```python
from build123d import *

# Parameters (mm, degrees)
SKETCH1_R           = 4.7625
BOSS_EXTRUDE1_DEPTH = 5.08
FILLET1_R           = 1.27


with BuildPart() as part:
    # Sketch1 → Boss-Extrude1 (new body)
    with BuildSketch(Plane.XY):
        Polygon((6.705982891, 2.965320691), (0.784948396, 7.290211886), (-5.921034494, 4.324891195), (-6.705982891, -2.965320691), (-0.784948396, -7.290211886), (5.921034494, -4.324891195), align=None)
        Circle(SKETCH1_R, mode=Mode.SUBTRACT)
    extrude(amount=BOSS_EXTRUDE1_DEPTH)

    # Fillet1
    fillet1_edges = [part.edges().sort_by_distance(p)[0] for p in [
        (-2.568043049, 5.807551541, 5.08),
        (-6.313508693, 0.679785252, 5.08),
        (-3.745465644, -5.127766289, 5.08),
        (2.568043049, -5.807551541, 5.08),
        (6.313508693, -0.679785252, 5.08),
        (3.745465644, 5.127766289, 5.08),
    ]]
    fillet(fillet1_edges, radius=FILLET1_R)


solid = part.part
```
The listing builds one solid part. Answer for the finished solid, in the listing's coordinates (mm). Give positions to 0.01 mm unless a question says otherwise; leave off trailing zeros. Order: outer loops, then holes, each group sorted by start corner. A loop starts at its lowest first (then second) coordinate and runs counter-clockwise, first axis right, second up. Notation, with made-up numbers: (-29, 43) - (10, 43) arc R15 cw to (10, 68) - close; hole circle Ø6 at (4, 42.25). An arc over 180 degrees is marked (long way). Answer in a Markdown table with one row per item. Add a question column.
Q1. The part is cut by section A-A (z = 3.4). Determine the outline of the cut face in (x, y) (1 decimal), then the cut area to 3 significant figures.
Q2. Find the intervals of material crossed by line 1 along Y through (x, z) = (0, 2.1); line 2 along X through (y, z) = (-1.25, 3.4); line 3 along Y through (x, z) = (4, 2.2), in increasing order. Write a range as [from, to].
Q3. Given P1, Ø1.5, axis at y = 2, z = 1.5, coming from the -X side; P2, Ø1.5, axis at y = -1.5, z = 2, coming from the -X side, each flat-ended and moving along its own axis, determine where each tip first touches the part or whether it passes through.
Q4. For a pull along Y with two mould halves and no side action, classify faces 1 (the flat face through (-2.52, 5.83, 1.88)), 2 (the cylindrical face through (-3.78, -2.9, 2.5)), 3 (the flat face through (-3.787, -5.097, 1.878)) as released by +Y, released by -Y, zero draft, split by the parting line, or undercut.
Determined:
| question | item | result |
|---|---|---|
| 1 | outline | (-6.7, -3) - (-0.8, -7.3) - (5.9, -4.3) - (6.7, 3) - (0.8, 7.3) - (-5.9, 4.3) - close; hole circle Ø9.5 at (0, 0) |
| 1 | area | 68.4 mm² |
| 2 | line 1 | y = [-6.94, -4.76], [4.76, 6.94] |
| 2 | line 2 | x = [-6.52, -4.6], [4.6, 6.25] |
| 2 | line 3 | y = [-5.17, -2.58], [2.58, 4.94] |
| 3 | P1 | stops at x = -6.25 |
| 3 | P2 | stops at x = -6.63 |
| 4 | face 1 | released by +Y |
| 4 | face 2 | undercut |
| 4 | face 3 | released by -Y |
